Read the model definition and answer for the solid it produces. Units are mm, in the model's axes. A direction names the side the tool comes from. Give positions to 0.01 mm unless a question says otherwise; leave off trailing zeros. Write each loop counter-clockwise with the first axis right and the second up, starting at its lowest first coordinate (ties: lowest second). Pieces come first, ordered by that corner, then holes. Notation, with made-up numbers: (-23, 46) -> (35, 46) arc R29 cw to (35, 70) -> close; hole circle Ø7 at (-28, -13). An arc over 180 degrees is marked (long way). Use a Markdown table: item, result.
from build123d import *

# Parameters (mm, degrees)
F0_W     = 400
F0_H     = 500
F0_W_2   = 50
F0_H_2   = 50
F1_DEPTH = 10
F2_W     = 30
F2_H     = 30
F2_R     = 5
F3_DEPTH = 25
F5_DEPTH = 190


with BuildPart() as f1:
    # F0 (on Top) → F1 (new body)
    with BuildSketch(Plane.XY):
        Rectangle(F0_W, F0_H)
        with Locations((0, -75)):
            Rectangle(F0_W_2, F0_H_2, mode=Mode.SUBTRACT)
        with Locations((0, 30)):
            Rectangle(F0_W_2, F0_H_2, mode=Mode.SUBTRACT)
    extrude(amount=F1_DEPTH)

    # F2 (on face) → F3 (join)
    with BuildSketch(Plane(origin=(0, 0, 0), x_dir=(1, 0, 0), z_dir=(0, 0, -1))):
        with Locations((160, 210)):
            Rectangle(F2_W, F2_H)
        with Locations((160, 210)):
            Circle(F2_R, mode=Mode.SUBTRACT)
        with Locations((160, -210)):
            Rectangle(F2_W, F2_H)
        with Locations((160, -210)):
            Circle(F2_R, mode=Mode.SUBTRACT)
        with Locations((-160, -210)):
            Rectangle(F2_W, F2_H)
        with Locations((-160, -210)):
            Circle(F2_R, mode=Mode.SUBTRACT)
        with Locations((-160, 210)):
            Rectangle(F2_W, F2_H)
        with Locations((-160, 210)):
            Circle(F2_R, mode=Mode.SUBTRACT)
    extrude(amount=F3_DEPTH)

    # F4 (on face) → F5 (join)
    with BuildSketch(Plane(origin=(0, 250, 0), x_dir=(-1, 0, 0), z_dir=(0, 1, 0))):
        Polygon((4, -20), (4, -8), (2, -8), (2, -18), (-9, -18), (-9, 0), (-26, 0), (-26, -2), (-11, -2), (-11, -20), align=None)
    extrude(amount=-F5_DEPTH)


solid = f1.part
Item 1: For a pull along X with two mould halves and no side action, classify faces 1 (the face through (-160, 225, -12)), 2 (the face through (-200, -3, 5)), 3 (the face through (-160, 210, 0)) as +X half, -X half, draft (parallel to the pull), parting line (faces both ways), or undercut.
Return value:
| item | result |
|---|---|
| face 1 | draft |
| face 2 | -X half |
| face 3 | undercut |
Item 2: Straight lines are drawn through the part: line 1 along X through (y, z) = (197, -7); line 2 along Y through (x, z) = (160, -17.5); line 3 along X through (y, z) = (-210, -10.25). For each, find the intervals that lie inside material, in ascending order. Write a range as [from, to].
Return value:
| item | result |
|---|---|
| line 1 | [-175, -145], [9, 11], [145, 175] |
| line 2 | [-225, -215], [-205, -195], [195, 205], [215, 225] |
| line 3 | [-175, -165], [-155, -145], [145, 155], [165, 175] |
Item 3: Each of these flat-tipped pins is pushed along its axis until it touches: P1, Ø8, axis at x = 160, y = -210, coming from the -Z side; P2, Ø7.5, axis at x = -154, z = -9.5, coming from the -Y side; P3, Ø5, axis at y = 93, z = -9.5, coming from the -X side; P4, Ø10, axis at y = -61.5, z = -7, coming from the +X side. Where does it stop, or does it pass through?
Return value:
| item | result |
|---|---|
| P1 | z = 0 |
| P2 | y = -225 |
| P3 | x = -4 |
| P4 | through |
Item 4: A cutting plane is placed at A-A (y = -80.5). Give the vertices of the cut face in (x, z), then the cut area to 3 significant figures.
Return value:
| item | result |
|---|---|
| outline | (-200, 0) -> (-25, 0) -> (-25, 10) -> (-200, 10) -> close; (25, 0) -> (200, 0) -> (200, 10) -> (25, 10) -> close |
| area | 3,500 mm^2 |
Item 5: A cutting plane is placed at B-B (y = 150.5). Give the vertices of the cut face in (x, z), then the cut area to 3 significant figures.
Return value:
| item | result |
|---|---|
| outline | (-200, 0) -> (9, 0) -> (9, -18) -> (-2, -18) -> (-2, -8) -> (-4, -8) -> (-4, -20) -> (11, -20) -> (11, -2) -> (26, -2) -> (26, 0) -> (200, 0) -> (200, 10) -> (-200, 10) -> close |
| area | 4,120 mm^2 |
Item 6: A cutting plane is placed at C-C (x = 62). Give the vertices of the cut face in (y, z).
Return value:
| item | result |
|---|---|
| outline | (-250, 0) -> (250, 0) -> (250, 10) -> (-250, 10) -> close |
Item 7: A tool of negligible diameter and unlimited length cuts with its end or side. For faces 4 (the face through (4, 156, -20)), 5 (the face through (3, 156, -18)), 6 (the face through (-160, 195, -12)), 7 (the face through (160, 210, 0)), from which of +Z, -Z, +X, -X, +Y, -Y can it reach the whole face along a straight path? Write none if from no direction.
Return value:
| item | result |
|---|---|
| face 4 | -Z, +Y, -Y |
| face 5 | +Y, -Y |
| face 6 | -Z, -X |
| face 7 | -Z |
Item 8: A cutting plane is placed at D-D (y = -22). Give the vertices of the cut face in (x, z), then the cut area to 3 significant figures.
Return value:
| item | result |
|---|---|
| outline | (-200, 0) -> (200, 0) -> (200, 10) -> (-200, 10) -> close |
| area | 4,000 mm^2 |
